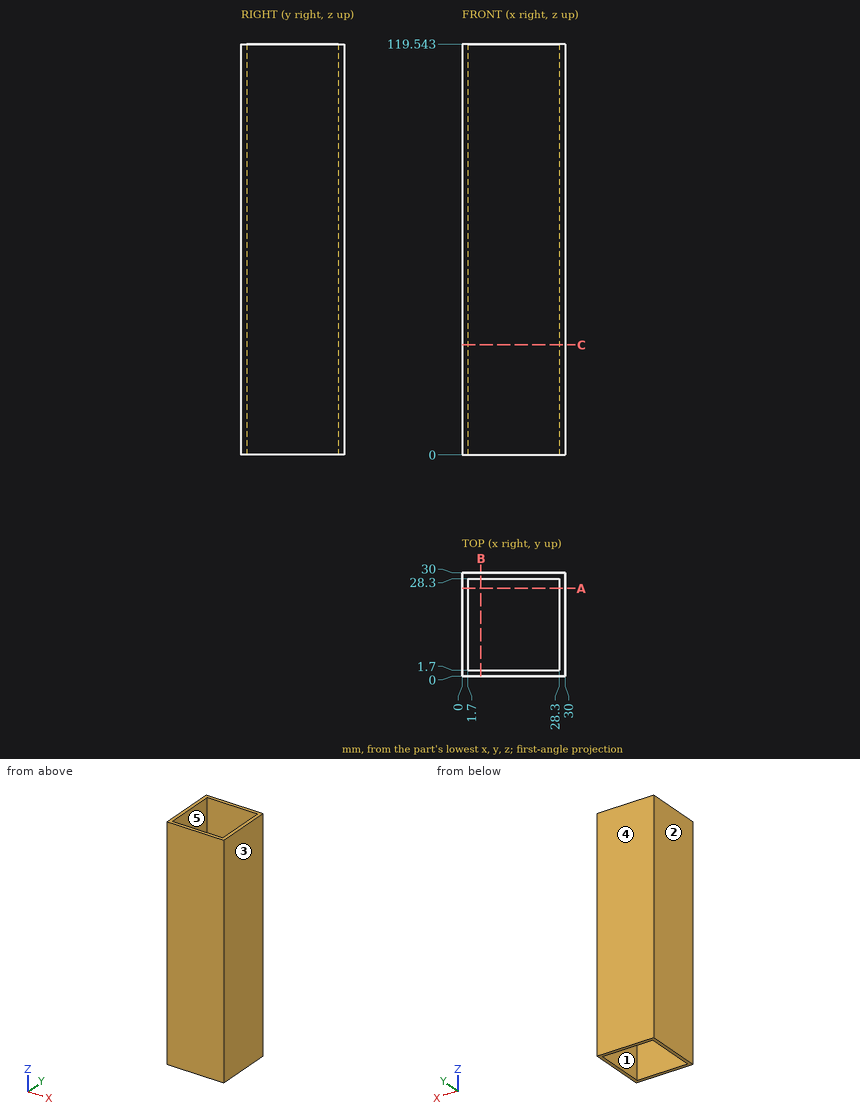
Verification items for this drawing (mm, ordinates from the low corner). A direction names the side the tool comes from. Coordinates: 2 decimals unless noted, no trailing zeros. Order: outer loops, then holes, each group sorted by start corner. A loop starts at its lowest first (then second) coordinate and runs counter-clockwise, first axis right, second up. Notation, with made-up numbers: M 12.5,-19 L 40.5,-19 A14 ccw 40.5,-6 Z; hole C 31.5,69 d2. An arc over 180 degrees is marked long. Answer as a JSON object with one key per item and string values.
Q1. Release check for a two-part mould opening along X. For the marked faces 1, 2 and 3 record: released by +X, released by -X, zero draft, split by the parting line, or undercut.
Results are:
{"face 1": "undercut", "face 2": "released by -X", "face 3": "released by +X"}
Q2. Scan line: line 1 (X direction, y = 27.5, z = 94). Record every from-to range of solid material in increasing order.
Results are:
{"line 1": "x = 0 to 1.7, 28.3 to 30"}
Q3. Depth check by flat-ended pin: pin 1 Ø4 at (x, y) = (5, 16.5) entering from -Z. Enter the tip coordinate at first touch or a pass-through.
Results are:
{"pin 1": "passes through"}
Q4. Tool access check on the marked faces 4 and 5. Record the directions out of +Z, -Z, +X, -X, +Y, -Y that give a thin tool (end or side, any length) a straight path to the whole face; none if there is none.
Results are:
{"face 4": "+Z, -Z, +X, -X, +Y", "face 5": "+Z, -Z"}
Q5. Cross-section at C-C on z = 32. Record the cut outline in (x, y).
Results are:
{"outline": "M 0,0 L 30,0 L 30,30 L 0,30 Z; hole M 1.7,1.7 L 28.3,1.7 L 28.3,28.3 L 1.7,28.3 Z"}
Q6. Cross-section at A-A on y = 25.5. Record the cut outline in (x, z), and give its area (3 significant figures).
Results are:
{"outline": "M 0,0 L 1.7,0 L 1.7,119.54 L 0,119.54 Z; M 28.3,0 L 30,0 L 30,119.54 L 28.3,119.54 Z", "area": "406 mm²"}
